Answer from the drawing. Dimensions are ordinates in mm from the lowest x, y and z of the part. A direction names the side the tool comes from. Round coordinates to 2 decimals unless told otherwise and drop trailing zeros. Loops run counter-clockwise (first coordinate to the right, second up) from the corner with the lowest first, then second, coordinate; pieces in that order, holes last. Notation, with made-up numbers: M 69.5,30.5 L 79.5,30.5 A18 ccw 79.5,53.5 Z; hole C 46,63 d7. An arc over 180 degrees is marked long. Answer as CSV lines item,"result".
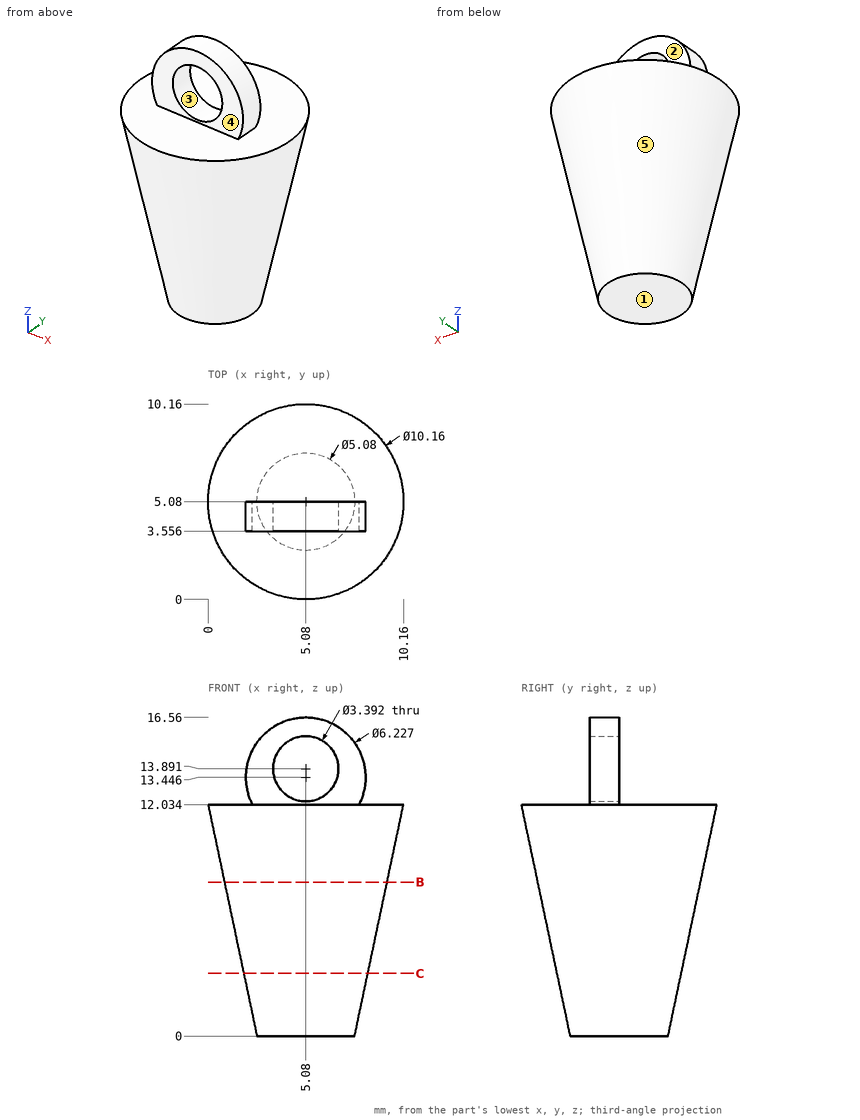
1) Each of these flat-tipped pins is pushed along its axis until it touches: P1, Ø1.5, axis at x = 9, y = 8, coming from the +Z side; P2, Ø2.5, axis at x = 6.5, z = 13.5, coming from the -Y side; P3, Ø5, axis at x = 4.5, z = 7.5, coming from the -Y side. Where does it stop, or does it pass through?
Evaluation:
P1,"stops at z = 12.03"
P2,"stops at y = 3.56"
P3,"stops at y = 0.44"
2) A tool of negligible diameter and unlimited length cuts with its end or side. For the marked faces 1 and 2, from which of +Z, -Z, +X, -X, +Y, -Y can it reach the whole face along a straight path? Write none if from no direction.
Evaluation:
face 1,"-Z, +X, -X, +Y, -Y"
face 2,"+Z, +X, -X, +Y"
3) Determine the mould class of the marked faces 3, 4 and 5 for opening direction Z: released by +Z, released by -Z, zero draft, split by the parting line, or undercut.
Evaluation:
face 3,"undercut"
face 4,"zero draft"
face 5,"released by -Z"
4) Straight lines are drawn through the part: line 1 (Z direction, x = 5.08, y = 4.4) (1 decimal); line 2 (Z direction, x = 6.75, y = 6); line 3 (Z direction, x = 6, y = 3.75) (1 decimal). For each, find the intervals that lie inside material, in ascending order.
Evaluation:
line 1,"z = 0 to 12.2, 15.6 to 16.6"
line 2,"z = 0 to 12.03"
line 3,"z = 0 to 12.5, 15.3 to 16.4"
5) Find section B-B, the plane z = 8. Give the vertices of the cut face in (x, y).
Evaluation:
outline,"C 5.08,5.08 d8.46"
6) Find section C-C, the plane z = 3.25. Give the vertices of the cut face in (x, y) (1 decimal).
Evaluation:
outline,"C 5.1,5.1 d6.5"
